Read the model definition and answer for the solid it produces. Units are mm, in the model's axes. Face numbers are marked on the shaded views. Coordinates: 2 decimals unless noted, no trailing zeros. Write each loop counter-clockwise with the first axis right and the second up, starting at its lowest first coordinate (ties: lowest second). Pieces come first, ordered by that corner, then holes. Notation, with made-up numbers: (35, 57.25) -> (50, 57.25) arc R14 ccw to (50, 69.25) -> close; hole circle Ø5 at (24.25, 81). An arc over 180 degrees is marked (long way). Answer in a Markdown table with one row per item. Add a question column.
Item 1: Section C-C on x = 1.45 is taken. Write down the section's boundary in (y, z) (1 decimal).
Item 2: Section B-B on z = 26 is taken. Write down the section's boundary in (x, y), then the cut area to 3 significant figures.
Item 3: Section A-A on y = 6.5 is taken. Write down the section's boundary in (x, z), then the cut area to 3 significant figures.
Item 4: Given pin 1 Ø6 at (y, z) = (-6.5, 10.5) entering from -X; pin 2 Ø1 at (x, y) = (1.5, -13) entering from -Z, each flat-ended and moving along its own axis, determine where each tip first touches the part or whether it passes through.
Item 5: For a pull along X with two mould halves and no side action, classify the marked faces 1 and 2 as +X half, -X half, draft (parallel to the pull), parting line (faces both ways), or undercut.
Item 6: Straight lines are drawn through the part: line 1 (Y direction, x = 0.25, z = -4); line 2 (Y direction, x = 0.75, z = 14); line 3 (Z direction, x = 2.3, y = 1). For each, find the intervals that lie inside material, in ascending order. Write a range as from..to.
Item 7: Section D-D on y = -5.5 is taken. Write down the section's boundary in (x, z), then the cut area to 3 significant figures.
Autodesk Inventor part; units mm, degrees
ref_plane "YZ Plane" through (0, 0, 0) normal (1, 0, 0) x (0, 1, 0)
ref_plane "XZ Plane" through (0, 0, 0) normal (0, 1, 0) x (-1, 0, 0)
ref_plane "XY Plane" through (0, 0, 0) normal (0, 0, 1) x (1, 0, 0)
sketch "スケッチ1" plane through (0, 0, 0) normal (1, 0, 0) x (0, 1, 0)
  line L0 (-4.615, 22.6143) -> (-8.3061, 28.9627)
  arc A0 (-8.3061, 28.9627) -> (3.9037, 31.3913) centre (3.0245, 3.9054) ccw
  line L1 (3.9037, 31.3913) -> (2.923, 24.1137)
  line L2 (2.923, 24.1137) -> (-4.615, 22.6143)
  circle A1 centre (3.0245, -5.0946) radius 1.7
  circle A2 centre (3.0245, 12.9054) radius 1.7
  circle A3 centre (3.0245, 3.9054) radius 5.2
  point P0 (0, 0)
extrude "押し出し1" add sketch "スケッチ1" along normal blind 2.5
properties part number "belt_liner_v1_3DP_P_F-1" material "ABS プラスチック"
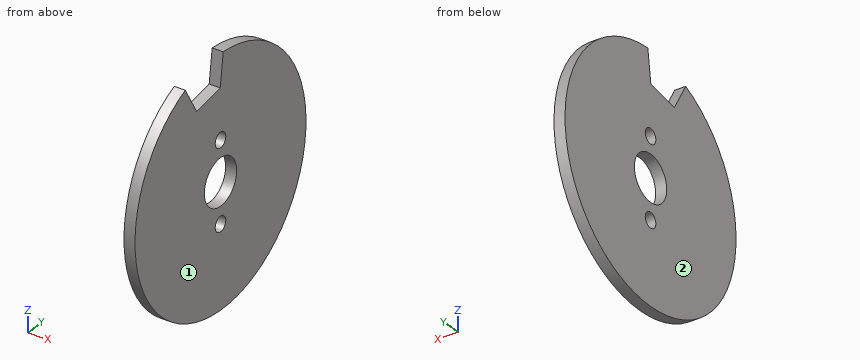
Results below:
| question | item | result |
|---|---|---|
| 1 | outline | (-8.3, 29) arc R27.5 ccw (long way) to (3.9, 31.4) -> (2.9, 24.1) -> (-4.6, 22.6) -> close; hole circle Ø10.4 at (3, 3.9); hole circle Ø3.4 at (3, -5.1); hole circle Ø3.4 at (3, 12.9) |
| 2 | outline | (0, -13.35) -> (2.5, -13.35) -> (2.5, -6.58) -> (0, -6.58) -> close; (0, 3.18) -> (2.5, 3.18) -> (2.5, 19.4) -> (0, 19.4) -> close |
| 2 | area | 57.5 mm2 |
| 3 | outline | (0, -23.37) -> (2.5, -23.37) -> (2.5, 0.04) -> (0, 0.04) -> close; (0, 7.77) -> (2.5, 7.77) -> (2.5, 31.18) -> (0, 31.18) -> close |
| 3 | area | 117 mm2 |
| 4 | pin 1 | stops at x = 0 |
| 4 | pin 2 | stops at z = -18.79 |
| 5 | face 1 | +X half |
| 5 | face 2 | -X half |
| 6 | line 1 | y = -23.31..1.72, 4.33..29.36 |
| 6 | line 2 | y = -22.56..1.72, 4.33..28.6 |
| 6 | line 3 | z = -23.52..-0.88, 8.7..23.73 |
| 7 | outline | (0, -22.24) -> (2.5, -22.24) -> (2.5, 24.14) -> (0, 24.14) -> close |
| 7 | area | 116 mm2 |
